Could you check a few things on this model? Use its own coordinates, in mm. A direction names the side the tool comes from. Coordinates: 2 decimals unless noted, no trailing zeros. Loops run counter-clockwise (first coordinate to the right, second up) from the corner with the lowest first, then second, coordinate; pieces in that order, holes last. Notation, with made-up numbers: M 40,37 L 59,37 A21 ccw 59,41 Z; hole C 80.25,-32 d2. An arc over 180 degrees is marked long. Return JSON: item names as keys, results as strings. Group by question number.
from build123d import *

# Parameters (mm, degrees)
SKETCH1_W                      = 101
SKETCH1_H                      = 37
BOSS_MAINBRIDGERIGHTHALF_DEPTH = 0.5
SKETCH2_W                      = 0.5
SKETCH2_H                      = 3
SKETCH2_H_2                    = 6
BOSS_METALTABS_DEPTH           = 9
SKETCH3_W                      = 0.6
SKETCH3_H                      = 8
CUT_EXTRUDE1_DEPTH             = 1.5


with BuildPart() as part:
    # Sketch1 → Boss-MainBridgeRightHalf (new body)
    with BuildSketch(Plane(origin=(0, 0, 0), x_dir=(1, 0, 0), z_dir=(0, 1, 0))):
        with Locations((50.5, 18.5)):
            Rectangle(SKETCH1_W, SKETCH1_H)
    boss_mainbridgerighthalf = extrude(amount=BOSS_MAINBRIDGERIGHTHALF_DEPTH)

    # Sketch2 → Boss-MetalTabs (add)
    with BuildSketch(Plane(origin=(0, 0.5, 0), x_dir=(1, 0, 0), z_dir=(0, 1, 0))):
        with Locations((100.75, 1.5)):
            Rectangle(SKETCH2_W, SKETCH2_H)
        with Locations((100.15, 28.5)):
            Rectangle(SKETCH2_W, SKETCH2_H_2)
        with Locations((100.15, 9)):
            Rectangle(SKETCH2_W, SKETCH2_H_2)
    boss_metaltabs = extrude(amount=BOSS_METALTABS_DEPTH)

    # Sketch3 → Cut-Extrude1 (cut, through all)
    with BuildSketch(Plane(origin=(0, 0.5, 0), x_dir=(1, 0, 0), z_dir=(0, 1, 0))):
        with Locations((100.7, 27.5)):
            Rectangle(SKETCH3_W, SKETCH3_H)
        with Locations((100.7, 8)):
            Rectangle(SKETCH3_W, SKETCH3_H)
    cut_extrude1 = extrude(amount=-CUT_EXTRUDE1_DEPTH, mode=Mode.SUBTRACT)

    # Mirror1: Boss-MainBridgeRightHalf, Boss-MetalTabs, Cut-Extrude1 across plane
    add(boss_mainbridgerighthalf.mirror(Plane(origin=(0, 0.5, 0), x_dir=(0, 0, 1), z_dir=(1, 0, 0))))
    add(boss_metaltabs.mirror(Plane(origin=(0, 0.5, 0), x_dir=(0, 0, 1), z_dir=(1, 0, 0))))
    add(cut_extrude1.mirror(Plane(origin=(0, 0.5, 0), x_dir=(0, 0, 1), z_dir=(1, 0, 0))), mode=Mode.SUBTRACT)


solid = part.part
(1) For faces 5 (the face through (-101, 5, -2)), 6 (the face through (-99.9, 5, -28)), which set-ups out of +Z, -Z, +X, -X, +Y, -Y let a thin tool reach every point of the face, with its end or its side?
(2) We'd pull the mould along X, two halves only. Please class faces 1 (the face through (99.9, 5, -28)), 2 (the face through (1, 0, -19)), 3 (the face through (99.9, 5, -9)), 4 (the face through (-100.4, 5, -9)): +X half, -X half, draft (parallel to the pull), parting line (faces both ways), or undercut.
(3) If I drill on L1, parallel to X at y = 5.5, z = -8.5; L2, parallel to Y at x = 84.5, z = -28, over which ranges is the centre line in solid material (lowest first)? Write a range as [from, to].
(4) Will these pins go through, and if not, where does the flat tip stop? P1, Ø1, axis at x = 76, y = 2, coming from the +Z side; P2, Ø3, axis at y = 3.5, z = -26, coming from the +X side; P3, Ø5, axis at x = 36.5, z = -15.5, coming from the -Y side; P4, Ø3, axis at y = 6.5, z = -9, coming from the -X side.
(5) Imagine slicing it at C-C, the plane x = -85. Write out the boundary of the cut face in (y, z).
(6) Imagine slicing it at A-A, the plane y = 5.75. Write out the boundary of the cut face in (x, z), then the cut area to 3 significant figures.
(7) Imagine slicing it at B-B, the plane z = -18. Write out the boundary of the cut face in (x, y), then the cut area to 3 significant figures.
Checks:
{
 "1": {"face 5": "+Z, -Z, -X, +Y, -Y", "face 6": "+Z, -Z, +Y"},
 "2": {"face 1": "undercut", "face 2": "draft", "face 3": "undercut", "face 4": "-X half"},
 "3": {"L1": "[-100.4, -99.9], [99.9, 100.4]", "L2": "[0, 0.5]"},
 "4": {"P1": "through", "P2": "x = 100.4", "P3": "y = 0", "P4": "x = -100.4"},
 "5": {"outline": "M 0,-37 L 0.5,-37 L 0.5,0 L 0,0 Z"},
 "6": {"outline": "M -101,-3 L -100.5,-3 L -100.5,0 L -101,0 Z; M -100.4,-31.5 L -99.9,-31.5 L -99.9,-25.5 L -100.4,-25.5 Z; M -100.4,-12 L -99.9,-12 L -99.9,-6 L -100.4,-6 Z; M 99.9,-31.5 L 100.4,-31.5 L 100.4,-25.5 L 99.9,-25.5 Z; M 99.9,-12 L 100.4,-12 L 100.4,-6 L 99.9,-6 Z; M 100.5,-3 L 101,-3 L 101,0 L 100.5,0 Z", "area": "15.0 mm²"},
 "7": {"outline": "M -101,0 L 101,0 L 101,0.5 L -101,0.5 Z", "area": "101 mm²"}
}
